Part print with two shaded views. Sizes in mm from the minimum x, y, z corner. Give positions to 0.01 mm unless a question says otherwise; leave off trailing zeros. Write each loop counter-clockwise with the first axis right and the second up, starting at its lowest first coordinate (ties: lowest second). Pieces come first, ordered by that corner, then holes.
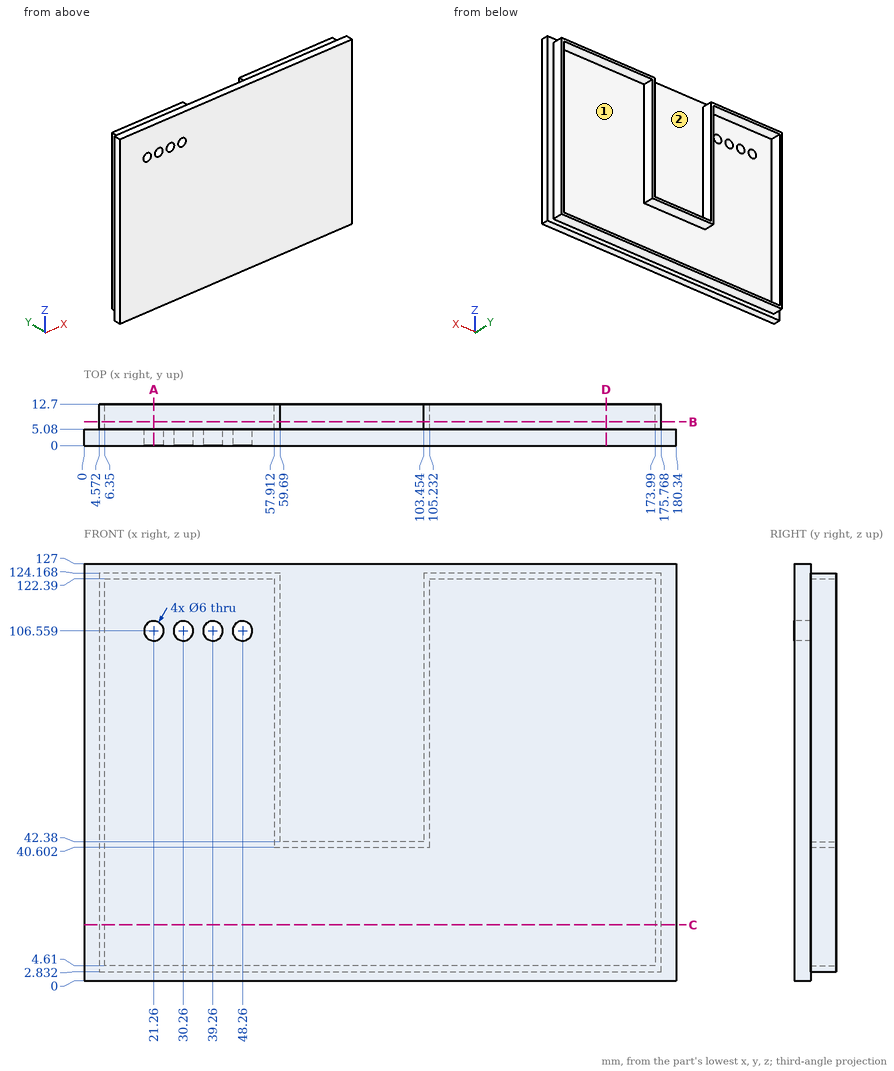
1) Saw through at B-B, the plane y = 7.25. Write the cut outline in (x, z), then the cut area to 3 significant figures.
Answers follow:
outline: (4.57, 2.83) - (175.77, 2.83) - (175.77, 124.17) - (103.45, 124.17) - (103.45, 42.38) - (59.69, 42.38) - (59.69, 124.17) - (4.57, 124.17) - close; hole (6.35, 4.61) - (173.99, 4.61) - (173.99, 122.39) - (105.23, 122.39) - (105.23, 40.6) - (57.91, 40.6) - (57.91, 122.39) - (6.35, 122.39) - close
area: 1,320 mm2
2) Saw through at D-D, the plane x = 159. Write the cut outline in (y, z), then the cut area to 3 significant figures.
Answers follow:
outline: (0, 0) - (5.08, 0) - (5.08, 2.83) - (12.7, 2.83) - (12.7, 4.61) - (5.08, 4.61) - (5.08, 122.39) - (12.7, 122.39) - (12.7, 124.17) - (5.08, 124.17) - (5.08, 127) - (0, 127) - close
area: 672 mm2
3) Saw through at C-C, the plane z = 17. Write the cut outline in (x, y).
Answers follow:
outline: (0, 0) - (180.34, 0) - (180.34, 5.08) - (175.77, 5.08) - (175.77, 12.7) - (173.99, 12.7) - (173.99, 5.08) - (6.35, 5.08) - (6.35, 12.7) - (4.57, 12.7) - (4.57, 5.08) - (0, 5.08) - close
4) Saw through at A-A, the plane x = 21.26. Write the cut outline in (y, z).
Answers follow:
outline: (0, 0) - (5.08, 0) - (5.08, 2.83) - (12.7, 2.83) - (12.7, 4.61) - (5.08, 4.61) - (5.08, 103.56) - (0, 103.56) - close; (0, 109.56) - (5.08, 109.56) - (5.08, 122.39) - (12.7, 122.39) - (12.7, 124.17) - (5.08, 124.17) - (5.08, 127) - (0, 127) - close
5) Two-plate mould, pull along Z, no slides. Class the marked faces 1 and 2: +Z half, -Z half, draft (parallel to the pull), parting line (faces both ways), or undercut.
Answers follow:
face 1: undercut
face 2: draft
6) Wall check: L1, parallel to X at y = 12.25, z = 51.5; L2, parallel to Z at x = 21.26, y = 3.5; L3, parallel to Z at x = 21.5, y = 9.5. Give the ranges that are in metal, low to high.
Answers follow:
L1: x = 4.57 to 6.35, 57.91 to 59.69, 103.45 to 105.23, 173.99 to 175.77
L2: z = 0 to 103.56, 109.56 to 127
L3: z = 2.83 to 4.61, 122.39 to 124.17
7) Pin check, flat tips, straight feed: pin 1 Ø4 at (x, y) = (144, 9.5) entering from -Z; pin 2 Ø1 at (x, z) = (147, 34) entering from -Y; pin 3 Ø4 at (x, y) = (92.5, 7.5) entering from +Z; pin 4 Ø6 at (x, y) = (23.5, 10) entering from +Z. Stop position of each tip, or through.
Answers follow:
pin 1: stops at z = 2.83
pin 2: stops at y = 0
pin 3: stops at z = 42.38
pin 4: stops at z = 124.17
